Source: CAD feature listing. Evaluate the final solid. Frame: model axes, mm. A direction names the side the tool comes from. Round coordinates to 2 decimals unless told otherwise and drop trailing zeros. Write each loop counter-clockwise with the first axis right and the second up, starting at its lowest first coordinate (ties: lowest second). Pieces come first, ordered by that corner, then holes. Notation, with made-up numbers: M 85,-27 L 144,-27 A5 cw 144,-23 Z; hole C 30.25,59.25 d7. An arc over 180 degrees is marked long. Answer in a Markdown table with one row per item. Add a question column.
Item 1: Set-up query: faces 1 (the face through (-0.651, 30.874, -5.043)), 2 (the face through (7.15, 10.14, -16.99)). Return all of +Z, -Z, +X, -X, +Y, -Y with unobstructed straight access to the full face (end or side cutting, diameter ignored); none if empty.
Item 2: Contact query for flat-ended pins moving along their axis: pin 1 (2 mm diameter, centred on x = 6, z = -4.5, fed in from +Y); pin 2 (1.5 mm diameter, centred on x = 0.5, y = 21, fed in from +Z). Output: stop coordinate, or through.
Item 3: Material intervals for probe 1 along Y at (x, z) = (-3.75, 0); probe 2 along Z at (x, y) = (-4, 19); probe 3 along Z at (x, y) = (-6, 19.5), sorted ascending.
Item 4: Cut plane B-B on z = -0.5. Return loops of the section in (x, y), and give its area (3 significant figures).
Item 5: Cut plane C-C on x = -8.5. Return loops of the section in (y, z).
Item 6: Cut plane D-D on y = 35.5. Return loops of the section in (x, z).
Autodesk Inventor part; units mm, degrees
ref_plane "YZ Plane" through (0, 0, 0) normal (1, 0, 0) x (0, 1, 0)
ref_plane "XZ Plane" through (0, 0, 0) normal (0, 1, 0) x (-1, 0, 0)
ref_plane "XY Plane" through (0, 0, 0) normal (0, 0, 1) x (1, 0, 0)
sketch "Schizzo1" plane through (0, 0, 0) normal (0, 1, 0) x (-1, 0, 0)
  line L0 (10, 20) -> (-10, 20)
  line L1 (-10, 20) -> (-10, -20)
  line L2 (-10, -20) -> (10, -20)
  line L3 (10, -20) -> (10, 20)
  line L4 (10, 20) -> (-10, -20) construction
  line L5 (-10, 20) -> (10, -20) construction
  point P0 (0, 0)
  dimension "d0" = 40
  dimension "d1" = 20
extrude "Estrusione1" add sketch "Schizzo1" along normal blind 20
sketch "Schizzo2" plane through (0, 20, 0) normal (0, 1, 0) x (1, 0, 0)
  line L0 (0, 0) -> (0, 10)
  circle A0 centre (0, 10) radius 5
  dimension "d4" = 10
  dimension "d5" = 10
extrude "Estrusione2" add sketch "Schizzo2" along normal blind 20
fillet "Raccordo1" radius 10 2 edges at (10, 10, -20) (-10, 10, -20)
fillet "Raccordo2" radius 2 1 edges at (-5, 20, -10)
properties part number "05-17-2023 cardine inferiore analisi fem"
Results below:
| question | item | result |
|---|---|---|
| 1 | face 1 | +Y |
| 1 | face 2 | -Z, +X, +Y, -Y |
| 2 | pin 1 | y = 20 |
| 2 | pin 2 | z = -3.99 |
| 3 | probe 1 | 0 to 20 |
| 3 | probe 2 | -19.17 to 20 |
| 3 | probe 3 | -18 to 20 |
| 4 | outline | M -10,0 L 10,0 L 10,20 L -10,20 Z |
| 4 | area | 400 mm2 |
| 5 | outline | M 0,-15.27 L 20,-15.27 L 20,20 L 0,20 Z |
| 6 | outline | C 0,-10 d10 |
